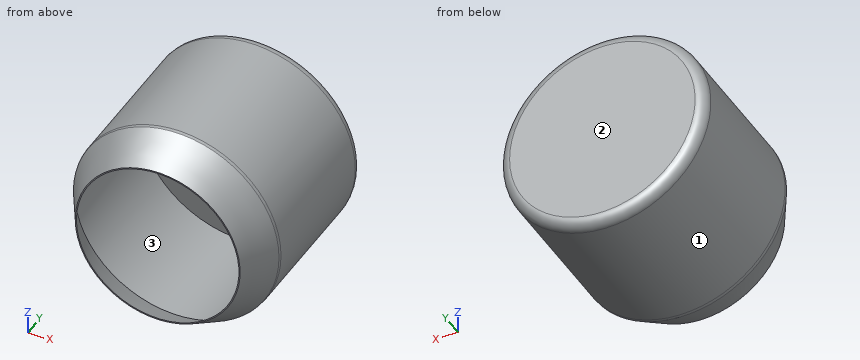
from build123d import *

# Parameters (mm, degrees)
F0_R     = 50
F1_DEPTH = 15
F2_R     = 50
F2_R_2   = 49.75
F3_DEPTH = 60
F6_R     = 5


# Not quite as in the source:
# - a fillet or chamfer that OpenCascade refuses, or shapes differently, is made with other operations: its cross-section is extruded or revolved along the edge and cut away or added


with BuildPart() as f1:
    # F0 (on Front) → F1 (new body)
    with BuildSketch(Plane.XZ):
        Circle(F0_R)
    extrude(amount=F1_DEPTH)

    # F2 (on face) → F3 (join)
    with BuildSketch(Plane.XZ.offset(15)):
        Circle(F2_R)
        Circle(F2_R_2, mode=Mode.SUBTRACT)
    extrude(amount=F3_DEPTH)

    # F4 (on Top) → F5 (revolve)
    with BuildSketch(Plane.XY):
        Polygon((-40, -92.0273140073), (-39.4221065602, -92.0273140073), (-49.289773818, -75), (-49.8676672578, -75), align=None)
    revolve(axis=Axis((0, -82.0273140073, 0), (0, -1, 0)))

    # F6
    f6_edges = [f1.edges().sort_by_distance(p)[0] for p in [
        (-50, 0, 0),
    ]]
    fillet(f6_edges, radius=F6_R)

    # F7: fillet of radius 10 on 1 edges, made by hand

    # F7_s1 → F7_t2 (revolve, cut)
    with BuildSketch(Plane.XY):
        with BuildLine():
            ThreePointArc((50, -73.378536806), (49.9668619078, -74.1919639453), (49.8676672578, -75))
            Line((49.8676672578, -75), (50, -75))
            Line((50, -75), (50, -73.378536806))
        make_face()
    revolve(axis=Axis((0, -75, 0), (0, -1, 0)), mode=Mode.SUBTRACT)


solid = f1.part
Can you work these out from the model? Positions are in its coordinate system, mm. Face numbers are marked on the shaded views. Round coordinates to 2 decimals unless told otherwise and drop trailing zeros. Order: outer loops, then holes, each group sorted by start corner. A loop starts at its lowest first (then second) coordinate and runs counter-clockwise, first axis right, second up. Notation, with made-up numbers: (70, 30.5) -> (95, 30.5) arc R13 ccw to (95, 41.5) -> close; hole circle Ø9 at (11.25, -36). An arc over 180 degrees is marked (long way). Write each question's results on one line, items separated by ' | '. Start each with the question number.
Item 1: If we section it at C-C, the plane x = 0: Write out the boundary of the cut face in (y, z), then the cut area to 3 significant figures.
Item 2: Thinking about a two-plate mould opening in X: for the marked faces 1, 2 and 3, which applies, +X half, -X half, draft (parallel to the pull), parting line (faces both ways), or undercut?
Item 3: Will these pins go through, and if not, where does the flat tip stop? pin 1 (1 mm diameter, centred on y = -28.5, z = 21.5, fed in from +X); pin 2 (6 mm diameter, centred on x = 28.5, z = -7.5, fed in from -Y); pin 3 (2 mm diameter, centred on y = -53.5, z = -19.5, fed in from -X).
Item 4: Please list where these lines run through material, in increasing order: L1, parallel to Z at x = 0, y = -61; L2, parallel to Y at x = -9, z = -36; L3, parallel to X at y = -81, z = 12.
Item 5: If we section it at B-B, the plane y = -16.5: Write out the boundary of the cut face in (x, z), then the cut area to 3 significant figures.
Item 6: If we section it at D-D, the plane y = -7: Write out the boundary of the cut face in (x, z).
Item 7: If we section it at A-A, the plane z = 0: Write out the boundary of the cut face in (x, y), then the cut area to 3 significant figures.
Results:
1) outline: (-92.03, -40) -> (-75, -49.87) arc R10 ccw to (-73.38, -50) -> (-5, -50) arc R5 ccw to (0, -45) -> (0, 45) arc R5 ccw to (-5, 50) -> (-73.38, 50) arc R10 ccw to (-75, 49.87) -> (-92.03, 40) -> (-92.03, 39.42) -> (-75, 49.29) -> (-75, 49.75) -> (-15, 49.75) -> (-15, -49.75) -> (-75, -49.75) -> (-75, -49.29) -> (-92.03, -39.42) -> close | area: 1,540 mm2
2) face 1: parting line | face 2: draft | face 3: undercut
3) pin 1: stops at x = 45.38 | pin 2: stops at y = -15 | pin 3: stops at x = -46.45
4) L1: z = -50 to -49.75, 49.75 to 50 | L2: y = -15 to 0 | L3: x = -44.81 to -44.21, 44.21 to 44.81
5) outline: circle Ø100 at (0, 0); hole circle Ø99.5 at (0, 0) | area: 78.3 mm2
6) outline: circle Ø100 at (0, 0)
7) outline: (-50, -73.38) arc R10 ccw to (-49.87, -75) -> (-40, -92.03) -> (-39.42, -92.03) -> (-49.29, -75) -> (-49.75, -75) -> (-49.75, -15) -> (49.75, -15) -> (49.75, -75) -> (49.29, -75) -> (39.42, -92.03) -> (40, -92.03) -> (49.87, -75) arc R10 ccw to (50, -73.38) -> (50, -5) arc R5 ccw to (45, 0) -> (-45, 0) arc R5 ccw to (-50, -5) -> close | area: 1,540 mm2
